Input: dimensioned drawing with shaded views. Units: mm. Origin: part minimum x, y, z. A direction names the side the tool comes from. Round coordinates to 2 decimals unless told otherwise and drop trailing zeros. Order: outer loops, then holes, each group sorted by start corner. A loop starts at its lowest first (then second) coordinate and runs counter-clockwise, first axis right, second up. Notation, with made-up numbers: M -39.75,69 L -35.75,69 A24 ccw -35.75,96 Z; hole C 5,30 d2. An arc over 180 degrees is marked long. Answer as CSV lines item,"result". Start each with the question number.
Item 1: Pull-direction query (X, two-part tool) for the marked faces 1, 2 and 3; classes: +X half, -X half, draft (parallel to the pull), parting line (faces both ways), or undercut.
Item 2: Section query C-C on y = 20. Return the cut outline in (x, z), plus the area to 3 significant figures.
Item 3: Section query D-D on z = 10. Return the cut outline in (x, y), plus the area to 3 significant figures.
Item 4: Set-up query: the marked faces 4, 5 and 6. Return all of +Z, -Z, +X, -X, +Y, -Y with unobstructed straight access to the full face (end or side cutting, diameter ignored); none if empty.
Item 5: First-contact query: P1, Ø2, axis at x = 13, z = 15.5, coming from the +Y side; P2, Ø1.5, axis at x = 26.5, z = 19.5, coming from the -Y side; P3, Ø4, axis at x = 80, y = 25, coming from the -Z side. Flat tips, straight axial feed; report the tip coordinate or a pass-through.
Item 6: Section query B-B on z = 20. Return the cut outline in (x, y).
Item 7: Line query: line 1 (Z direction, x = 89, y = 20); line 2 (X direction, y = 10.5, z = 33); line 3 (X direction, y = 13, z = 38). Output: solid intervals per line, ascending. Write a range as [from, to].
Item 8: Section query A-A on x = 53.5. Return the cut outline in (y, z), plus the area to 3 significant figures.
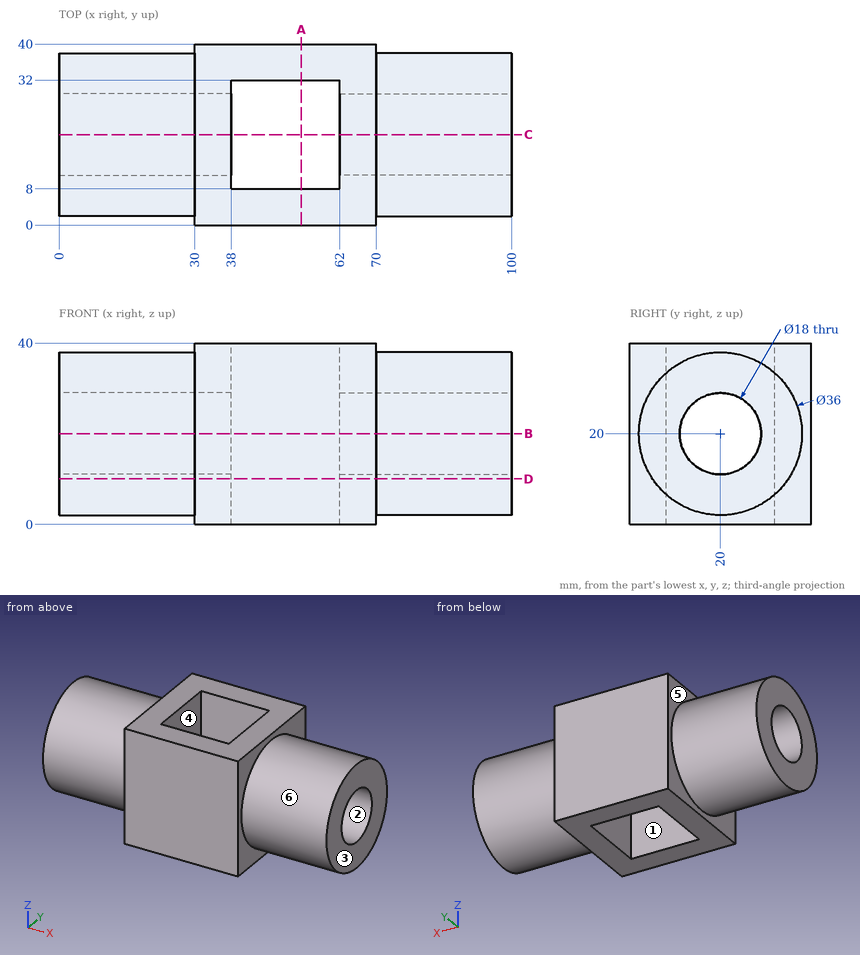
Results:
1,face 1,"undercut"
1,face 2,"draft"
1,face 3,"+X half"
2,outline,"M 0,2 L 30,2 L 30,0 L 38,0 L 38,11 L 0,11 Z; M 0,29 L 38,29 L 38,40 L 30,40 L 30,38 L 0,38 Z; M 62,0 L 70,0 L 70,2 L 100,2 L 100,11 L 62,11 Z; M 62,29 L 100,29 L 100,38 L 70,38 L 70,40 L 62,40 Z"
2,area,"1,430 mm^2"
3,outline,"M 0,5.03 L 30,5.03 L 30,0 L 70,0 L 70,5.03 L 100,5.03 L 100,34.97 L 70,34.97 L 70,40 L 30,40 L 30,34.97 L 0,34.97 Z; hole M 38,8 L 62,8 L 62,32 L 38,32 Z"
3,area,"2,820 mm^2"
4,face 4,"+Z, -Z"
4,face 5,"-X"
4,face 6,"+X"
5,P1,"y = 37.66"
5,P2,"y = 2"
5,P3,"z = 2.25"
6,outline,"M 0,2 L 30,2 L 30,0 L 70,0 L 70,2 L 100,2 L 100,11 L 62,11 L 62,8 L 38,8 L 38,11 L 0,11 Z; M 0,29 L 38,29 L 38,32 L 62,32 L 62,29 L 100,29 L 100,38 L 70,38 L 70,40 L 30,40 L 30,38 L 0,38 Z"
7,line 1,"[2, 11], [29, 38]"
7,line 2,"[0, 38], [62, 100]"
7,line 3,"[30, 38], [62, 70]"
8,outline,"M 0,0 L 8,0 L 8,40 L 0,40 Z; M 32,0 L 40,0 L 40,40 L 32,40 Z"
8,area,"640 mm^2"
